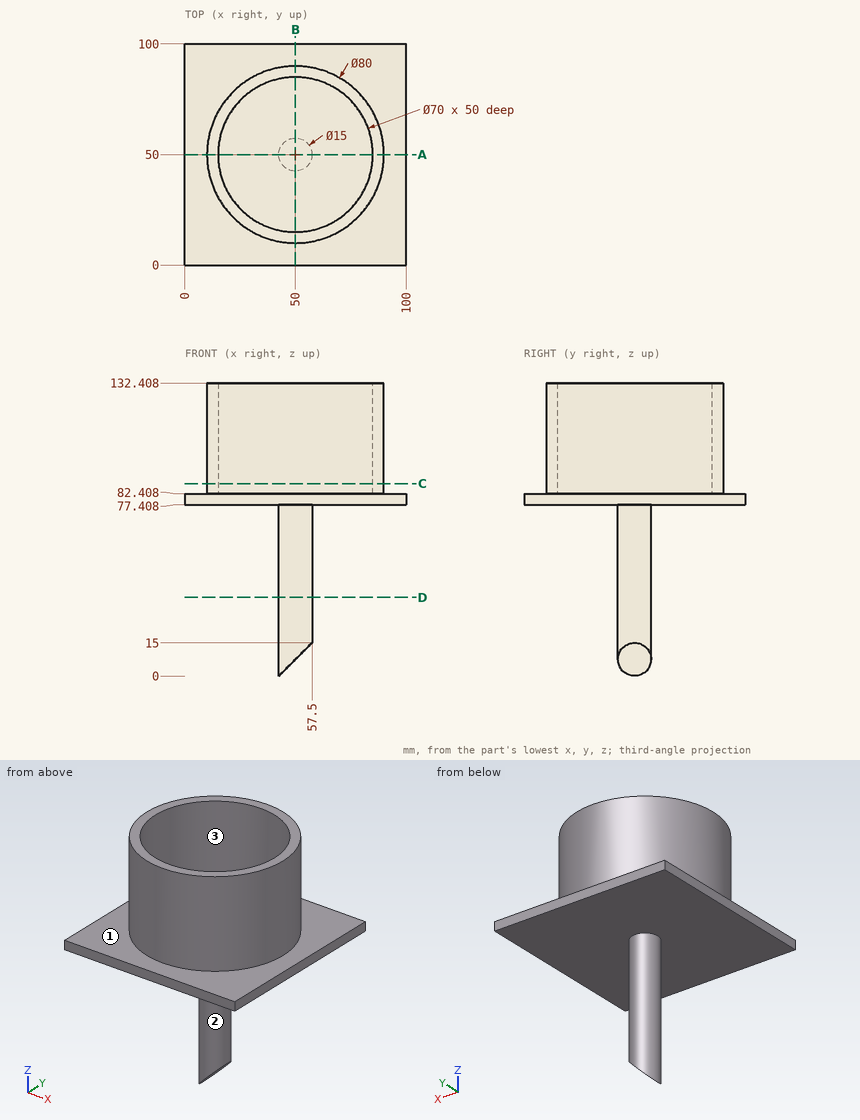
Print and shaded views of the part. All mm, measured from the part's lowest x, y and z. Round coordinates to 2 decimals unless told otherwise and drop trailing zeros. Order: outer loops, then holes, each group sorted by start corner. A loop starts at its lowest first (then second) coordinate and runs counter-clockwise, first axis right, second up.
Q1. Two-plate mould, pull along X, no slides. Class the marked faces 1, 2 and 3: pulls with the +X half, pulls with the -X half, needs draft (parallel to the pull), parting line crosses it, or undercut.
Q2. Slice it at D-D (z = 35.5). Write the cut outline in (x, y).
Q3. Slice it at C-C (z = 87). Write the cut outline in (x, y), and give its area (3 significant figures).
Q4. Wall check: L1, parallel to Y at x = 50, z = 120; L2, parallel to Z at x = 93, y = 11.5; L3, parallel to Z at x = 52.5, y = 43. Give the ranges that are in metal, low to high.
Q5. Slice it at A-A (y = 50). Write the cut outline in (x, z), and give its area (3 significant figures).
Q6. Slice it at B-B (x = 50). Write the cut outline in (y, z), and give its area (3 significant figures).
Q7. Drop flat-ended pins along their axis: pin 1 (1.5 mm diameter, centred on x = 80.5, z = 117, fed in from +Y); pin 2 (6 mm diameter, centred on x = 79.5, z = 95.5, fed in from +Y); pin 3 (10 mm diameter, centred on y = 57.5, z = 100, fed in from +X). Give the stop position or say it passes through.
Results below:
1. face 1: needs draft
1. face 2: parting line crosses it
1. face 3: undercut
2. outline: circle Ø15 at (50, 50)
3. outline: circle Ø80 at (50, 50); hole circle Ø70 at (50, 50)
3. area: 1,180 mm2
4. L1: y = 10 to 15, 85 to 90
4. L2: z = 77.41 to 82.41
4. L3: z = 10 to 82.41
5. outline: (0, 77.41) - (42.5, 77.41) - (42.5, 0) - (57.5, 15) - (57.5, 77.41) - (100, 77.41) - (100, 82.41) - (90, 82.41) - (90, 132.41) - (85, 132.41) - (85, 82.41) - (15, 82.41) - (15, 132.41) - (10, 132.41) - (10, 82.41) - (0, 82.41) - close
5. area: 2,050 mm2
6. outline: (0, 77.41) - (42.5, 77.41) - (42.5, 7.5) - (57.5, 7.5) - (57.5, 77.41) - (100, 77.41) - (100, 82.41) - (90, 82.41) - (90, 132.41) - (85, 132.41) - (85, 82.41) - (15, 82.41) - (15, 132.41) - (10, 132.41) - (10, 82.41) - (0, 82.41) - close
6. area: 2,050 mm2
7. pin 1: stops at y = 76.74
7. pin 2: stops at y = 79.96
7. pin 3: stops at x = 89.92
